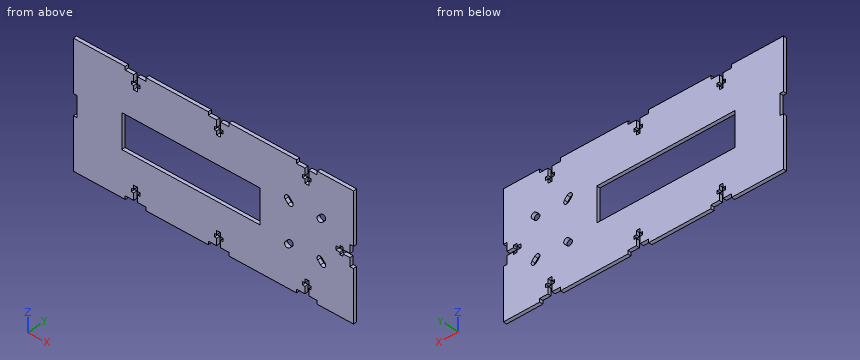
from build123d import *

# Parameters (mm, degrees)
BOSS_EXTRUDE1_DEPTH = 2.54
CUT_EXTRUDE1_REACH  = 4.54
CUT_EXTRUDE2_REACH  = 4.54
SKETCH4_W           = 101.6
SKETCH4_H           = 25.4


with BuildPart() as part:
    # Sketch2 → Boss-Extrude1 (new body)
    with BuildSketch(Plane(origin=(0, 0, 0), x_dir=(1, 0, 0), z_dir=(0, 1, 0))):
        Polygon((-102.87, -45.72), (-64.77, -45.72), (-64.77, -43.18), (-58.5978, -43.18), (-58.5978, -38.1), (-60.325, -38.1), (-60.325, -35.66795), (-58.5978, -35.66795), (-58.5978, -32.766), (-55.7022, -32.766), (-55.7022, -35.66795), (-53.975, -35.66795), (-53.975, -38.1), (-55.7022, -38.1), (-55.7022, -43.18), (-49.53, -43.18), (-49.53, -45.72), (-3.81, -45.72), (-3.81, -43.18), (2.3622, -43.18), (2.3622, -38.1), (0.635, -38.1), (0.635, -35.66795), (2.3622, -35.66795), (2.3622, -32.766), (5.2578, -32.766), (5.2578, -35.66795), (6.985, -35.66795), (6.985, -38.1), (5.2578, -38.1), (5.2578, -43.18), (11.43, -43.18), (11.43, -45.72), (60.96, -45.72), (60.96, -43.18), (67.1322, -43.18), (67.1322, -38.1), (65.405, -38.1), (65.405, -35.66795), (67.1322, -35.66795), (67.1322, -32.766), (70.0278, -32.766), (70.0278, -35.66795), (71.755, -35.66795), (71.755, -38.1), (70.0278, -38.1), (70.0278, -43.18), (76.2, -43.18), (76.2, -45.72), (102.87, -45.72), (102.87, -7.62), (100.33, -7.62), (100.33, -1.4478), (95.25, -1.4478), (95.25, -3.175), (92.81795, -3.175), (92.81795, -1.4478), (89.916, -1.4478), (89.916, 1.4478), (92.81795, 1.4478), (92.81795, 3.175), (95.25, 3.175), (95.25, 1.4478), (100.33, 1.4478), (100.33, 7.62), (102.87, 7.62), (102.87, 45.72), (76.2, 45.72), (76.2, 43.18), (70.0278, 43.18), (70.0278, 38.1), (71.755, 38.1), (71.755, 35.66795), (70.0278, 35.66795), (70.0278, 32.766), (67.1322, 32.766), (67.1322, 35.66795), (65.405, 35.66795), (65.405, 38.1), (67.1322, 38.1), (67.1322, 43.18), (60.96, 43.18), (60.96, 45.72), (11.43, 45.72), (11.43, 43.18), (5.2578, 43.18), (5.2578, 38.1), (6.985, 38.1), (6.985, 35.66795), (5.2578, 35.66795), (5.2578, 32.766), (2.3622, 32.766), (2.3622, 35.66795), (0.635, 35.66795), (0.635, 38.1), (2.3622, 38.1), (2.3622, 43.18), (-3.81, 43.18), (-3.81, 45.72), (-49.53, 45.72), (-49.53, 43.18), (-55.7022, 43.18), (-55.7022, 38.1), (-53.975, 38.1), (-53.975, 35.66795), (-55.7022, 35.66795), (-55.7022, 32.766), (-58.5978, 32.766), (-58.5978, 35.66795), (-60.325, 35.66795), (-60.325, 38.1), (-58.5978, 38.1), (-58.5978, 43.18), (-64.77, 43.18), (-64.77, 45.72), (-102.87, 45.72), (-102.87, 7.62), (-100.33, 7.62), (-100.33, -7.62), (-102.87, -7.62), align=None)
    extrude(amount=-BOSS_EXTRUDE1_DEPTH)

    # Sketch3 → Cut-Extrude1 (cut, up to next)
    with BuildSketch(Plane(origin=(0, 0, 0), x_dir=(1, 0, 0), z_dir=(0, 1, 0)), mode=Mode.PRIVATE) as cut_extrude1_sk1:
        with BuildLine():
            Line((81.873223588, 14.562666667), (79.841223588, 12.290821602))
            ThreePointArc((79.841223588, 12.290821602), (76.792666667, 12.120931347), (76.622776412, 15.169488268))
            Line((76.622776412, 15.169488268), (78.654776412, 17.441333333))
            ThreePointArc((78.654776412, 17.441333333), (81.703333333, 17.611223588), (81.873223588, 14.562666667))
        make_face()
    cut_extrude1_tool1 = extrude(cut_extrude1_sk1.sketch, amount=-CUT_EXTRUDE1_REACH, mode=Mode.PRIVATE) & part.part
    add(cut_extrude1_tool1.solids().sort_by_distance((79.248, 0, -14.866077))[0], mode=Mode.SUBTRACT)
    # Sketch3 → Cut-Extrude1 (cut, up to next)
    with BuildSketch(Plane(origin=(0, 0, 0), x_dir=(1, 0, 0), z_dir=(0, 1, 0)), mode=Mode.PRIVATE) as cut_extrude1_sk2:
        with BuildLine():
            Line((52.746776412, 14.562666667), (54.778776412, 12.290821602))
            ThreePointArc((54.778776412, 12.290821602), (57.827333333, 12.120931347), (57.997223588, 15.169488268))
            Line((57.997223588, 15.169488268), (55.965223588, 17.441333333))
            ThreePointArc((55.965223588, 17.441333333), (52.916666667, 17.611223588), (52.746776412, 14.562666667))
        make_face()
    cut_extrude1_tool2 = extrude(cut_extrude1_sk2.sketch, amount=-CUT_EXTRUDE1_REACH, mode=Mode.PRIVATE) & part.part
    add(cut_extrude1_tool2.solids().sort_by_distance((55.372, 0, -14.866077))[0], mode=Mode.SUBTRACT)
    # Sketch3 → Cut-Extrude1 (cut, up to next)
    with BuildSketch(Plane(origin=(0, 0, 0), x_dir=(1, 0, 0), z_dir=(0, 1, 0)), mode=Mode.PRIVATE) as cut_extrude1_sk3:
        with BuildLine():
            Line((81.873223588, -14.562666667), (79.841223588, -12.290821602))
            ThreePointArc((79.841223588, -12.290821602), (76.792666667, -12.120931347), (76.622776412, -15.169488268))
            Line((76.622776412, -15.169488268), (78.654776412, -17.441333333))
            ThreePointArc((78.654776412, -17.441333333), (81.703333333, -17.611223588), (81.873223588, -14.562666667))
        make_face()
    cut_extrude1_tool3 = extrude(cut_extrude1_sk3.sketch, amount=-CUT_EXTRUDE1_REACH, mode=Mode.PRIVATE) & part.part
    add(cut_extrude1_tool3.solids().sort_by_distance((79.248, 0, 14.866077))[0], mode=Mode.SUBTRACT)
    # Sketch3 → Cut-Extrude1 (cut, up to next)
    with BuildSketch(Plane(origin=(0, 0, 0), x_dir=(1, 0, 0), z_dir=(0, 1, 0)), mode=Mode.PRIVATE) as cut_extrude1_sk4:
        with BuildLine():
            Line((52.746776412, -14.562666667), (54.778776412, -12.290821602))
            ThreePointArc((54.778776412, -12.290821602), (57.827333333, -12.120931347), (57.997223588, -15.169488268))
            Line((57.997223588, -15.169488268), (55.965223588, -17.441333333))
            ThreePointArc((55.965223588, -17.441333333), (52.916666667, -17.611223588), (52.746776412, -14.562666667))
        make_face()
    cut_extrude1_tool4 = extrude(cut_extrude1_sk4.sketch, amount=-CUT_EXTRUDE1_REACH, mode=Mode.PRIVATE) & part.part
    add(cut_extrude1_tool4.solids().sort_by_distance((55.372, 0, 14.866077))[0], mode=Mode.SUBTRACT)

    # Sketch4 → Cut-Extrude2 (cut, up to next)
    with BuildSketch(Plane(origin=(0, 0, 0), x_dir=(1, 0, 0), z_dir=(0, 1, 0)), mode=Mode.PRIVATE) as cut_extrude2_sk1:
        with Locations((-16.51, 0)):
            Rectangle(SKETCH4_W, SKETCH4_H)
    cut_extrude2_tool1 = extrude(cut_extrude2_sk1.sketch, amount=-CUT_EXTRUDE2_REACH, mode=Mode.PRIVATE) & part.part
    add(cut_extrude2_tool1.solids().sort_by_distance((-16.51, 0, 0))[0], mode=Mode.SUBTRACT)


solid = part.part
Model file for the job. Use its own axes, mm. Give positions to 0.01 mm unless a question says otherwise; leave off trailing zeros. Write each loop counter-clockwise with the first axis right and the second up, starting at its lowest first coordinate (ties: lowest second). Pieces come first, ordered by that corner, then holes. Notation, with made-up numbers: M 60,-2.75 L 79,-2.75 A13 ccw 79,21.25 Z; hole C 10,89 d10. An arc over 180 degrees is marked long. One line per item, written item: value. Start each with the question number.
Q1. Saw through at B-B, the plane y = -1.3. State how many separate pieces and enclosed holes the cut face has, plus the area to 3 significant figures.
Q2. Saw through at A-A, the plane x = -32.5. Write the cut outline in (y, z).
Q3. Probe probe 1 along Z at (x, y) = (65.5, -2.2); probe 2 along X at (y, z) = (-1.7, 33.5); probe 3 along Z at (x, y) = (-38, -0.5). List the from-to ranges inside material, lowest first. Write a range as [from, to].
Q4. Drop flat-ended pins along their axis: pin 1 Ø8 at (x, z) = (-62, 3.5) entering from -Y; pin 2 Ø0.8 at (x, y) = (8, -1.5) entering from -Z; pin 3 Ø1.3 at (x, y) = (-62, -1.5) entering from +Z; pin 4 Ø0.9 at (y, z) = (-1.5, -2) entering from +X. Give the stop position or say it passes through.
Output values:
1. separate pieces: 1
1. enclosed holes: 5
1. area: 15,500 mm²
2. outline: M -2.54,-45.72 L 0,-45.72 L 0,-12.7 L -2.54,-12.7 Z; M -2.54,12.7 L 0,12.7 L 0,45.72 L -2.54,45.72 Z
3. probe 1: z = [-43.18, -38.1], [-35.67, 35.67], [38.1, 43.18]
3. probe 2: x = [-102.87, -58.6], [-55.7, 2.36], [5.26, 67.13], [70.03, 102.87]
3. probe 3: z = [-45.72, -12.7], [12.7, 45.72]
4. pin 1: passes through
4. pin 2: stops at z = -43.18
4. pin 3: stops at z = 43.18
4. pin 4: stops at x = 100.33
